from build123d import *

# Parameters (mm, degrees)
ESQUISSE1_W             = 85
ESQUISSE1_H             = 56
ESQUISSE1_R             = 1
BOSS_EXTRU_1_DEPTH      = 1
ESQUISSE2_W             = 6
ESQUISSE2_H             = 15.454409224
ESQUISSE2_W_2           = 8
ESQUISSE2_H_2           = 4.146304914
BOSS_EXTRU_2_DEPTH      = 30
CONG_1_R                = 5
ESQUISSE3_R             = 0.85
ENL_V_MAT_EXTRU_1_DEPTH = 5


with BuildPart() as part:
    # Esquisse1 → Boss.-Extru.1 (new body)
    with BuildSketch(Plane(origin=(0, 0, 0), x_dir=(1, 0, 0), z_dir=(0, 1, 0))):
        with Locations((9.925986842, -10.804276316)):
            Rectangle(ESQUISSE1_W, ESQUISSE1_H)
        with Locations(Location((-29.074013158, 13.695723684, 0), (0, 0, 270))):
            Circle(ESQUISSE1_R, mode=Mode.SUBTRACT)
        with Locations(Location((28.925986842, 13.695723684, 0), (0, 0, 270))):
            Circle(ESQUISSE1_R, mode=Mode.SUBTRACT)
        with Locations(Location((29.363486842, -35.304276316, 0), (0, 0, 270))):
            Circle(ESQUISSE1_R, mode=Mode.SUBTRACT)
        with Locations(Location((-29.074013158, -35.304276316, 0), (0, 0, 270))):
            Circle(ESQUISSE1_R, mode=Mode.SUBTRACT)
    extrude(amount=BOSS_EXTRU_1_DEPTH)

    # Esquisse2 → Boss.-Extru.2 (add)
    with BuildSketch(Plane.XZ):
        with Locations((-6.574013158, 10.804276316)):
            Rectangle(ESQUISSE2_W, ESQUISSE2_H)
        with Locations((20.05121001, 10.804276316)):
            Rectangle(ESQUISSE2_W_2, ESQUISSE2_H_2)
    extrude(amount=BOSS_EXTRU_2_DEPTH)

    # Congé1
    cong_1_edges = [part.edges().sort_by_distance(p)[0] for p in [
        (-9.574013158, 0, 10.804276316),
        (-6.574013158, 0, 3.077071704),
        (-3.574013158, 0, 10.804276316),
        (-6.574013158, 0, 18.531480928),
        (16.05121001, 0, 10.804276316),
        (20.05121001, 0, 8.731123859),
        (24.05121001, 0, 10.804276316),
        (20.05121001, 0, 12.877428773),
    ]]
    fillet(cong_1_edges, radius=CONG_1_R)

    # Esquisse3 → Enlèv. mat.-Extru.1 (cut)
    with BuildSketch(Plane.XZ.offset(30)):
        with Locations(Location((-6.574013158, 14.304276316, 0), (0, 0, 270))):
            Circle(ESQUISSE3_R)
        with Locations(Location((-6.574013158, 7.304276316, 0), (0, 0, 270))):
            Circle(ESQUISSE3_R)
    extrude(amount=-ENL_V_MAT_EXTRU_1_DEPTH, mode=Mode.SUBTRACT)


solid = part.part
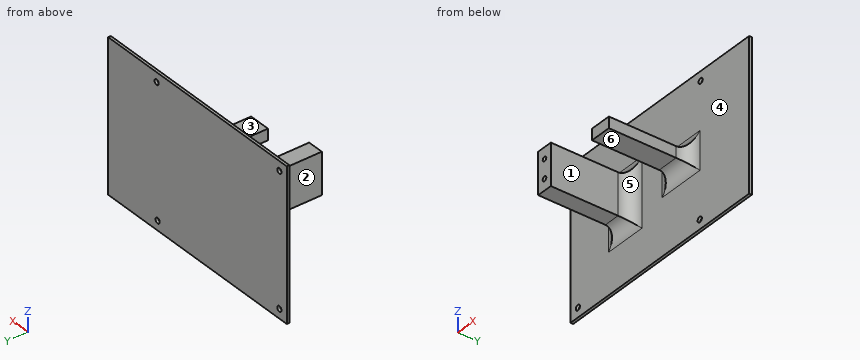
CAD build for the part. Positions are in the model's coordinates, mm. Face numbers are marked on the shaded views. A direction names the side the tool comes from. Coordinates: 2 decimals unless noted, no trailing zeros. Write each loop counter-clockwise with the first axis right and the second up, starting at its lowest first coordinate (ties: lowest second). Pieces come first, ordered by that corner, then holes. Notation, with made-up numbers: M 24,58 L 35,58 A24 cw 35,79 Z; hole C 81,75.5 d10. An arc over 180 degrees is marked long. Return JSON: item names as keys, results as strings.
Item 1: Slice it at D-D, the plane z = -0.5. Write the cut outline in (x, y).
Findings below:
{"outline": "M -32.57,0 L -14.57,0 A5 cw -13.15,-0.21 L 0,-0.21 A5 cw 1.43,0 L 52.43,0 L 52.43,1 L -32.57,1 Z"}
Item 2: Two-plate mould, pull along X, no slides. Class the marked faces 1, 2 and 3: +X half, -X half, draft (parallel to the pull), parting line (faces both ways), or undercut.
Findings below:
{"face 1": "undercut", "face 2": "-X half", "face 3": "draft"}
Item 3: Which spindle directions (+Z, -Z, +X, -X, +Y, -Y) get a long thin tool onto all of the face, cutting with end or side? Do the marked faces 4, 5 and 6. Say none if no direction does.
Findings below:
{"face 4": "-Y", "face 5": "+Z, -Z, -Y", "face 6": "-Z, +X, -Y"}
Item 4: Slice it at C-C, the plane x = 10. Write the cut outline in (y, z), and give its area (3 significant figures).
Findings below:
{"outline": "M 0,-17.2 L 1,-17.2 L 1,38.8 L 0,38.8 Z", "area": "56.0 mm2"}
Item 5: Slice it at A-A, the plane y = -6. Write the cut outline in (x, z).
Findings below:
{"outline": "M -9.57,3.08 L -3.57,3.08 L -3.57,18.53 L -9.57,18.53 Z; M 16.05,8.73 L 24.05,8.73 L 24.05,12.88 L 16.05,12.88 Z"}
Item 6: Probe line 1 (Y direction, x = -17.5, z = 33.5); line 2 (Z direction, x = -5.5, y = -16); line 3 (Z direction, x = 20.5, y = -8). List the from-to ranges inside material, lowest first. Write a range as from..to.
Findings below:
{"line 1": "y = 0..1", "line 2": "z = 3.08..18.53", "line 3": "z = 8.73..12.88"}
Item 7: Drop flat-ended pins along their axis: pin 1 Ø12.5 at (y, z) = (-11.5, 10) entering from -X; pin 2 Ø0.8 at (x, z) = (-6.5, 14.5) entering from -Y; pin 3 Ø6 at (y, z) = (-8, 23.5) entering from -X; pin 4 Ø2.5 at (x, z) = (28.93, -13.7) entering from -Y. Give the stop position or say it passes through.
Findings below:
{"pin 1": "stops at x = -9.57", "pin 2": "stops at y = -25", "pin 3": "passes through", "pin 4": "stops at y = 0"}
Item 8: Slice it at B-B, the plane z = 11.5. Write the cut outline in (x, y).
Findings below:
{"outline": "M -32.57,0 L -14.57,0 A5 cw -9.57,-5 L -9.57,-30 L -3.57,-30 L -3.57,-5 A5 cw 1.43,0 L 11.05,0 A5 cw 16.05,-5 L 16.05,-30 L 24.05,-30 L 24.05,-5 A5 cw 29.05,0 L 52.43,0 L 52.43,1 L -32.57,1 Z"}
